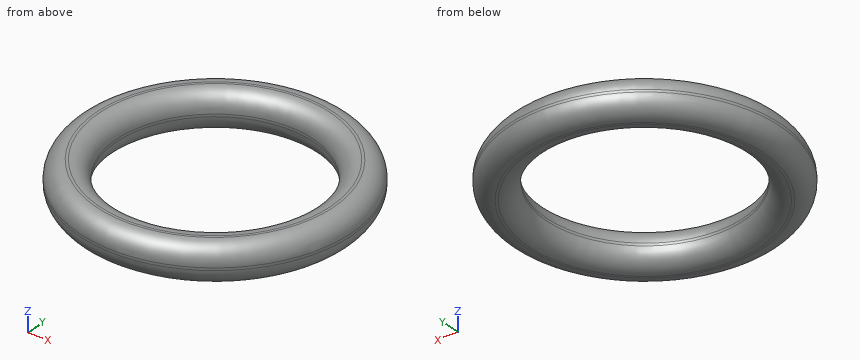
```python
from build123d import *

# Parameters (mm, degrees)
CYLINDER_R        = 7.85
CYLINDER_DEPTH    = 10
CYLINDER001_R     = 10.85
CYLINDER001_DEPTH = 3
FILLET_R          = 1.4


with BuildPart() as cylinder:
    # Cylinder → Cylinder (new body)
    with BuildSketch(Plane(origin=(7, 0, 0), x_dir=(1, 0, 0), z_dir=(0, 0, 1))):
        Circle(CYLINDER_R)
    extrude(amount=CYLINDER_DEPTH)


with BuildPart() as fillet_body:
    # Cylinder001 → Cylinder001 (new body)
    with BuildSketch(Plane(origin=(7, 0, 0), x_dir=(1, 0, 0), z_dir=(0, 0, 1))):
        Circle(CYLINDER001_R)
    extrude(amount=CYLINDER001_DEPTH)

    # Cut: cut Cylinder
    add(cylinder.part, mode=Mode.SUBTRACT)

    # Fillet
    fillet_edges = [fillet_body.edges().sort_by_distance(p)[0] for p in [
        (-3.85, 0, 3),
        (-3.85, 0, 0),
        (-0.85, 0, 3),
        (-0.85, 0, 0),
    ]]
    fillet(fillet_edges, radius=FILLET_R)


with BuildPart() as fillet_body_1:
    # Fillet placement: moved
    add(fillet_body.part.moved(Location((13, 0, 0))))


solid = fillet_body_1.part
```
Input: part model. Units: mm. Frame: model coordinates. Round coordinates to 2 decimals unless told otherwise and drop trailing zeros. Write each loop counter-clockwise with the first axis right and the second up, starting at its lowest first coordinate (ties: lowest second). Pieces come first, ordered by that corner, then holes. Notation, with made-up numbers: M 74,14 L 112,14 A18 cw 112,20 Z; hole C 65.5,-17 d9. An arc over 180 degrees is marked long. Write each question's results on one line, items separated by ' | '.
Q1. Section query A-A (x = 20). Return loops of the section in (y, z), and give its area (3 significant figures).
Results:
outline: M -10.85,1.4 A1.4 ccw -9.45,0 L -9.25,0 A1.4 ccw -7.85,1.4 L -7.85,1.6 A1.4 ccw -9.25,3 L -9.45,3 A1.4 ccw -10.85,1.6 Z; M 7.85,1.4 A1.4 ccw 9.25,0 L 9.45,0 A1.4 ccw 10.85,1.4 L 10.85,1.6 A1.4 ccw 9.45,3 L 9.25,3 A1.4 ccw 7.85,1.6 Z | area: 14.6 mm^2
Q2. Section query C-C (z = 2). Return loops of the section in (x, y).
Results:
outline: C 20,0 d21.58; hole C 20,0 d15.82
Q3. Pin query (flat end, axial travel): P1, Ø10, axis at x = 17.5, y = 1, coming from the +Z side; P2, Ø1.5, axis at y = 3.5, z = 1, coming from the -X side; P3, Ø1, axis at x = 23.5, z = 2, coming from the +Y side; P4, Ø1, axis at x = 24, z = 1, coming from the +Y side. Return the tip coordinate at first contact, or that it passes through.
Results:
P1: passes through | P2: stops at x = 9.52 | P3: stops at y = 10.4 | P4: stops at y = 10.24
Q4. Section query D-D (z = 0.3). Return loops of the section in (x, y), and give its area (3 significant figures).
Results:
outline: C 20,0 d20.63; hole C 20,0 d16.77 | area: 114 mm^2
Q5. Section query B-B (y = 0). Return loops of the section in (x, z), and give its area (3 significant figures).
Results:
outline: M 9.15,1.4 A1.4 ccw 10.55,0 L 10.75,0 A1.4 ccw 12.15,1.4 L 12.15,1.6 A1.4 ccw 10.75,3 L 10.55,3 A1.4 ccw 9.15,1.6 Z; M 27.85,1.4 A1.4 ccw 29.25,0 L 29.45,0 A1.4 ccw 30.85,1.4 L 30.85,1.6 A1.4 ccw 29.45,3 L 29.25,3 A1.4 ccw 27.85,1.6 Z | area: 14.6 mm^2
Q6. Line query: line 1 along Y through (x, z) = (20, 1.5); line 2 along X through (y, z) = (0.75, 1.3); line 3 along Y through (x, z) = (20.75, 2.8). Output: solid intervals per line, ascending.
Results:
line 1: y = -10.85 to -7.85, 7.85 to 10.85 | line 2: x = 9.18 to 12.18, 27.82 to 30.82 | line 3: y = -10.14 to -8.5, 8.5 to 10.14
